Read the model definition and answer for the solid it produces. Units are mm, in the model's axes. A direction names the side the tool comes from. Coordinates: 2 decimals unless noted, no trailing zeros. Write each loop counter-clockwise with the first axis right and the second up, starting at its lowest first coordinate (ties: lowest second). Pieces come first, ordered by that corner, then holes. Notation, with made-up numbers: (-38, 87) -> (-7, 87) arc R21 cw to (-7, 113) -> close; hole circle Ø2 at (73, 1). An arc over 180 degrees is marked (long way). Return JSON: item names as keys, results as strings.
from build123d import *

# Parameters (mm, degrees)
SKETCH_R        = 2.4
SKETCH_R_2      = 10
PAD_DEPTH       = 4.5
SKETCH001_R     = 12
SKETCH001_R_2   = 6.1
PAD001_DEPTH    = 4
SKETCH002_R     = 7
SKETCH002_R_2   = 4
PAD002_DEPTH    = 12
FILLET_R        = 1
CHAMFER_SIZE    = 1
CHAMFER001_SIZE = 0.5


with BuildPart() as part:
    # Sketch → Pad (new body)
    with BuildSketch(Plane.XY):
        with BuildLine():
            ThreePointArc((12.172496, -5.837838), (13.5, 0), (12.172496, 5.837838))
            Line((4.959165, 20.878378), (12.172496, 5.837838))
            ThreePointArc((4.959165, 20.878378), (0, 24), (-4.959165, 20.878378))
            Line((-12.172496, 5.837838), (-4.959165, 20.878378))
            ThreePointArc((-12.172496, 5.837838), (-13.5, 0), (-12.172496, -5.837838))
            Line((-4.959165, -20.878378), (-12.172496, -5.837838))
            ThreePointArc((-4.959165, -20.878378), (0, -24), (4.959165, -20.878378))
            Line((4.959165, -20.878378), (12.172496, -5.837838))
        make_face()
        with Locations((0, 18.5)):
            Circle(SKETCH_R, mode=Mode.SUBTRACT)
        with Locations((0, -18.5)):
            Circle(SKETCH_R, mode=Mode.SUBTRACT)
        Circle(SKETCH_R_2, mode=Mode.SUBTRACT)
    extrude(amount=PAD_DEPTH)

    # Sketch001 (on Face13 of Pad) → Pad001 (join)
    with BuildSketch(Plane.XY.offset(4.5)):
        Circle(SKETCH001_R)
        Circle(SKETCH001_R_2, mode=Mode.SUBTRACT)
    extrude(amount=PAD001_DEPTH)

    # Sketch002 → Pad002 (join)
    with BuildSketch(Plane.XY.offset(0.5)):
        Circle(SKETCH002_R)
        Circle(SKETCH002_R_2, mode=Mode.SUBTRACT)
    extrude(amount=PAD002_DEPTH)

    # Fillet
    fillet_edges = [part.edges().sort_by_distance(p)[0] for p in [
        (-8.56583, -13.358108, 4.5),
        (-13.5, 0, 4.5),
        (-8.56583, 13.358108, 4.5),
        (0, 24, 4.5),
        (8.56583, 13.358108, 4.5),
        (8.56583, -13.358108, 4.5),
        (0, -24, 4.5),
        (13.5, 0, 4.5),
    ]]
    fillet(fillet_edges, radius=FILLET_R)

    # Chamfer
    chamfer_edges = [part.edges().sort_by_distance(p)[0] for p in [
        (-7, 0, 12.5),
    ]]
    chamfer(chamfer_edges, length=CHAMFER_SIZE)

    # Chamfer001
    chamfer001_edges = [part.edges().sort_by_distance(p)[0] for p in [
        (-12, 0, 8.5),
    ]]
    chamfer(chamfer001_edges, length=CHAMFER001_SIZE)


solid = part.part
1. A tool of negligible diameter and unlimited length cuts with its end or side. For faces 4 (the face through (-8.616, 13.253, 1.726)), 5 (the face through (-2.17, -9.76, 2.22)), 6 (the face through (-11.99, 0.53, 6.23)), from which of +Z, -Z, +X, -X, +Y, -Y can it reach the whole face along a straight path? Write none if from no direction.
Taken from the geometry:
{"face 4": "+Z, -Z, -X, +Y", "face 5": "-Z", "face 6": "+Z"}
2. The part is cut by section A-A (z = 2.75). Determine the outline of the cut face in (x, y), then the cut area to 3 significant figures.
Taken from the geometry:
{"outline": "(-12.17, -5.84) -> (-4.96, -20.88) arc R5.5 ccw to (4.96, -20.88) -> (12.17, -5.84) arc R13.5 ccw to (12.17, 5.84) -> (4.96, 20.88) arc R5.5 ccw to (-4.96, 20.88) -> (-12.17, 5.84) arc R13.5 ccw to start; circle Ø14 at (0, 0); hole circle Ø20 at (0, 0); hole circle Ø8 at (0, 0); hole circle Ø4.8 at (0, -18.5); hole circle Ø4.8 at (0, 18.5)", "area": "618 mm2"}
3. Consider L1, parallel to Y at x = 0, z = 2.1; L2, parallel to Y at x = 1.25, z = 2.25; L3, parallel to Y at x = 0, z = 8. Determine where each line is inside the solid, lowest interval first.
Taken from the geometry:
{"L1": "y = -24 to -20.9, -16.1 to -10, -7 to -4, 4 to 7, 10 to 16.1, 20.9 to 24", "L2": "y = -23.86 to -20.55, -16.45 to -9.92, -6.89 to -3.8, 3.8 to 6.89, 9.92 to 16.45, 20.55 to 23.86", "L3": "y = -12 to -4, 4 to 12"}
4. Flat-ended cylindrical pins translate along their axes: pin 1 Ø9 at (x, y) = (0, 0) entering from -Z; pin 2 Ø3 at (x, y) = (7, 4.5) entering from +Z; pin 3 Ø5 at (x, z) = (-10, 3.5) entering from -Y. Find the tip coordinate at first contact, or state that the pin passes through.
Taken from the geometry:
{"pin 1": "stops at z = 0.5", "pin 2": "stops at z = 11.68", "pin 3": "stops at y = -15.58"}
5. The part is cut by section D-D (z = 6.5). Determine the outline of the cut face in (x, y), then the cut area to 3 significant figures.
Taken from the geometry:
{"outline": "circle Ø24 at (0, 0); hole circle Ø8 at (0, 0)", "area": "402 mm2"}
6. For a pull along Y with two mould halves and no side action, classify faces 1 (the face through (8.515, 13.463, 1.726)), 2 (the face through (-8.515, -13.463, 1.726)), 3 (the face through (-0.52, -20.843, 2.218)) as +Y half, -Y half, draft (parallel to the pull), parting line (faces both ways), or undercut.
Taken from the geometry:
{"face 1": "+Y half", "face 2": "-Y half", "face 3": "undercut"}
7. The part is cut by section C-C (x = 0). Count the separate pieces of the cut face and the enclosed holes in it, then the cut area to 3 significant figures.
Taken from the geometry:
{"separate pieces": "4", "enclosed holes": "0", "area": "193 mm2"}
